from build123d import *

# Parameters (mm, degrees)
SKETCH2_R             = 6
CUT_EXTRUDE1_DEPTH    = 43.213741838
HOLE_WIZARD_M41_D     = 4.5
HOLE_WIZARD_M41_DEPTH = 22
HOLE_WIZARD_M41_TIP   = 1.351936393
CHAMFER1_SIZE         = 0.5


with BuildPart() as part:
    # Sketch1 → Revolve1 (revolve)
    with BuildSketch(Plane.XY, mode=Mode.PRIVATE) as revolve1_sk:
        Polygon((0, 0), (-21, 0), (-21, 6), (-10.5, 6), (-10.5, 30), (0, 30), align=None)
    revolve(revolve1_sk.sketch.rotate(Axis((0, 0, 0), (0, 1, 0)), 270), axis=Axis((0, 0, 0), (0, 1, 0)))

    # Sketch2 → Cut-Extrude1 (cut, through all)
    with BuildSketch(Plane.XZ):
        with Locations(Location((0, 0, 0), (0, 0, 270))):
            Circle(SKETCH2_R)
    extrude(amount=-CUT_EXTRUDE1_DEPTH, mode=Mode.SUBTRACT)

    # Отверстие с зазором M41
    with Locations(Plane(origin=(0, 6, 0), x_dir=(1, 0, 0), z_dir=(0, 1, 0))):
        with Locations((0, 16), (16, 0), (0, -16), (-16, 0)):
            Hole(HOLE_WIZARD_M41_D / 2, depth=HOLE_WIZARD_M41_DEPTH)
            with Locations((0, 0, -(HOLE_WIZARD_M41_DEPTH + HOLE_WIZARD_M41_TIP / 2))):  # 118° drill point
                Cone(0, HOLE_WIZARD_M41_D / 2, HOLE_WIZARD_M41_TIP, mode=Mode.SUBTRACT)

    # Chamfer1
    chamfer1_edges = [part.edges().sort_by_distance(p)[0] for p in [
        (0, 30, 10.5),
        (0, 6, 21),
        (0, 0, 21),
    ]]
    chamfer(chamfer1_edges, length=CHAMFER1_SIZE)


solid = part.part
Verification items for the finished model (mm, model axes). Give positions to 0.01 mm unless a question says otherwise; leave off trailing zeros. Write each loop counter-clockwise with the first axis right and the second up, starting at its lowest first coordinate (ties: lowest second). Pieces come first, ordered by that corner, then holes. Notation, with made-up numbers: (49, 10.5) -> (57, 10.5) arc R20 cw to (57, 16.5) -> close; hole circle Ø2 at (6, -28). An arc over 180 degrees is marked (long way). Use CSV: the item, a comma, the result in double quotes.
(1) Material ranges on L1, parallel to X at y = 22.5, z = 0; L2, parallel to X at y = 11.5, z = 1.5; L3, parallel to Y at x = -15, z = 11.5, recorded low to high.
Derived:
L1,"x = -10.5 to -6, 6 to 10.5"
L2,"x = -10.39 to -5.81, 5.81 to 10.39"
L3,"y = 0 to 6"
(2) Sectioned sample at B-B (y = 4.5). Record the cut outline in (x, z), plus the area to 3 significant figures.
Derived:
outline,"circle Ø42 at (0, 0); hole circle Ø4.5 at (-16, 0); hole circle Ø12 at (0, 0); hole circle Ø4.5 at (0, -16); hole circle Ø4.5 at (0, 16); hole circle Ø4.5 at (16, 0)"
area,"1,210 mm^2"
(3) Sectioned sample at C-C (y = 26.5). Record the cut outline in (x, z), plus the area to 3 significant figures.
Derived:
outline,"circle Ø21 at (0, 0); hole circle Ø12 at (0, 0)"
area,"233 mm^2"
(4) Release check for a two-part mould opening along Z. For faces 1 (the cylindrical face through (0.488, 2.958, -13.804)), 2 (the cylindrical face through (-3.2, 17.9, -10)), 3 (the flat face through (9, 6, -9)) record: +Z half, -Z half, draft (parallel to the pull), parting line (faces both ways), or undercut.
Derived:
face 1,"undercut"
face 2,"parting line"
face 3,"draft"
(5) Go/stop test with flat-tipped pins: pin 1 (1 mm diameter, centred on x = -8, z = -3.5, fed in from -Y); pin 2 (4 mm diameter, centred on y = 12, z = 0.5, fed in from +X); pin 3 (7 mm diameter, centred on x = 16, z = 0, fed in from +Y); pin 4 (8 mm diameter, centred on x = -2, y = 14.5, fed in from -Z). Record where each tip stops, or that it passes through.
Derived:
pin 1,"stops at y = 0"
pin 2,"stops at x = 10.5"
pin 3,"stops at y = 6"
pin 4,"stops at z = -10.5"
(6) Sectioned sample at A-A (x = 0). Record the cut outline in (y, z).
Derived:
outline,"(0, -20.5) -> (0.5, -21) -> (5.5, -21) -> (6, -20.5) -> (6, -18.25) -> (0, -18.25) -> close; (0, -13.75) -> (6, -13.75) -> (6, -10.5) -> (29.5, -10.5) -> (30, -10) -> (30, -6) -> (0, -6) -> close; (0, 6) -> (30, 6) -> (30, 10) -> (29.5, 10.5) -> (6, 10.5) -> (6, 13.75) -> (0, 13.75) -> close; (0, 18.25) -> (6, 18.25) -> (6, 20.5) -> (5.5, 21) -> (0.5, 21) -> (0, 20.5) -> close"
